Model file for the job. Use its own axes, mm. Face numbers are marked on the shaded views. Coordinates: 2 decimals unless noted, no trailing zeros. Write each loop counter-clockwise with the first axis right and the second up, starting at its lowest first coordinate (ties: lowest second). Pieces come first, ordered by that corner, then holes. Notation, with made-up numbers: M 28.25,11 L 40.25,11 A21 ccw 40.25,22 Z; hole C 68.5,48 d10. An arc over 180 degrees is marked long. Put each result on its own line as item: value. Start each with the question number.
Q1. Cut at A-A (z = 2.6). Write the cut outline in (x, y), then the cut area to 3 significant figures.
Q2. Drill centre lines: line 1 along Y through (x, z) = (2.25, 4.25); line 2 along Y through (x, z) = (-1.25, 1.95); line 3 along X through (y, z) = (0.5, 1.1). Where is each one in solid material? Low to high.
Q3. Pull direction Y, two halves, no side cores. Call the marked faces 1, 2 and 3: pulls with the +Y half, pulls with the -Y half, needs draft (parallel to the pull), parting line crosses it, or undercut.
Q4. Drop flat-ended pins along their axis: pin 1 (1.5 mm diameter, centred on x = -1.5, y = 4, fed in from -Z); pin 2 (3 mm diameter, centred on x = 0, z = 2.5, fed in from +Y); pin 3 (3 mm diameter, centred on x = -3.5, z = 1.5, fed in from -Y). Give the stop position or say it passes through.
```python
from build123d import *

# Parameters (mm, degrees)
SKETCH1_R           = 3
BOSS_EXTRUDE1_DEPTH = 5.2


with BuildPart() as part:
    # Sketch1 → Boss-Extrude1 (new body)
    with BuildSketch(Plane.XY):
        Polygon((0, 5.773502692), (-5, 2.886751346), (-5, -2.886751346), (0, -5.773502692), (5, -2.886751346), (5, 2.886751346), align=None)
        Circle(SKETCH1_R, mode=Mode.SUBTRACT)
    extrude(amount=BOSS_EXTRUDE1_DEPTH)

    # Sketch2 → Cut-Revolve2 (revolve, cut)
    with BuildSketch(Plane(origin=(0, 0, 0), x_dir=(0, 0, -1), z_dir=(0, 1, 0))):
        Polygon((-4.396152423, -8), (-6.405771366, -0.5), (-6.405771366, -8), align=None)
    cut_revolve2 = revolve(axis=Axis((0, 0, -2.80878951), (0, 0, 1)), mode=Mode.SUBTRACT)

    # Mirror1: Cut-Revolve2 across plane
    add(cut_revolve2.mirror(Plane.XY.offset(2.6)), mode=Mode.SUBTRACT)


solid = part.part
```
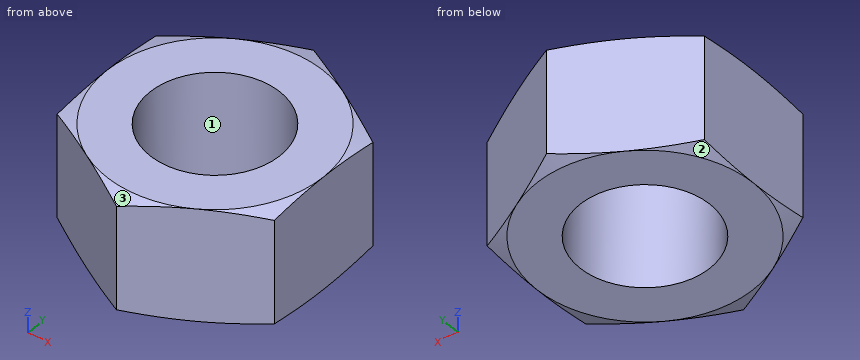
Computed values:
1. outline: M -5,-2.89 L 0,-5.77 L 5,-2.89 L 5,2.89 L 0,5.77 L -5,2.89 Z; hole C 0,0 d6
1. area: 58.3 mm2
2. line 1: -4.47 to -1.98, 1.98 to 4.47
2. line 2: -5.05 to -2.73, 2.73 to 5.05
2. line 3: -5 to -2.96, 2.96 to 5
3. face 1: undercut
3. face 2: pulls with the +Y half
3. face 3: pulls with the -Y half
4. pin 1: z = 0
4. pin 2: y = 5.77
4. pin 3: y = -4.62
